```python
from build123d import *

# Parameters (mm, degrees)
CYLINDER_R        = 8
CYLINDER_DEPTH    = 5
CYLINDER001_R     = 2.5
CYLINDER001_DEPTH = 10
CHAMFER_SIZE      = 0.2
SKETCH_R          = 7.171484
SKETCH_R_2        = 3.208205
POCKET_DEPTH      = 0.3
SKETCH001_R       = 7.114293
SKETCH001_R_2     = 3.634589
POCKET001_DEPTH   = 0.3
CHAMFER001_SIZE   = 0.1


with BuildPart() as part:
    # Cylinder → Cylinder (join)
    with BuildSketch(Plane.XY):
        Circle(CYLINDER_R)
    extrude(amount=CYLINDER_DEPTH)

    # Cylinder001 → Cylinder001 (cut)
    with BuildSketch(Plane.XY):
        Circle(CYLINDER001_R)
    extrude(amount=CYLINDER001_DEPTH, mode=Mode.SUBTRACT)

    # Chamfer
    chamfer_edges = [part.edges().sort_by_distance(p)[0] for p in [
        (-8, 0, 5),
        (-8, 0, 0),
        (-2.5, 0, 5),
        (-2.5, 0, 0),
    ]]
    chamfer(chamfer_edges, length=CHAMFER_SIZE)

    # Sketch (on Face5 of Chamfer) → Pocket (cut)
    with BuildSketch(Plane.XY.offset(5)):
        Circle(SKETCH_R)
        Circle(SKETCH_R_2, mode=Mode.SUBTRACT)
    extrude(amount=-POCKET_DEPTH, mode=Mode.SUBTRACT)

    # Sketch001 (on Face4 of Pocket) → Pocket001 (cut)
    with BuildSketch(Plane(origin=(0, 0, 0), x_dir=(1, 0, 0), z_dir=(0, 0, -1))):
        Circle(SKETCH001_R)
        Circle(SKETCH001_R_2, mode=Mode.SUBTRACT)
    extrude(amount=-POCKET001_DEPTH, mode=Mode.SUBTRACT)

    # Chamfer001
    chamfer001_edges = [part.edges().sort_by_distance(p)[0] for p in [
        (-7.171484, 0, 5),
        (-7.114293, 0, 0),
    ]]
    chamfer(chamfer001_edges, length=CHAMFER001_SIZE)


solid = part.part
```
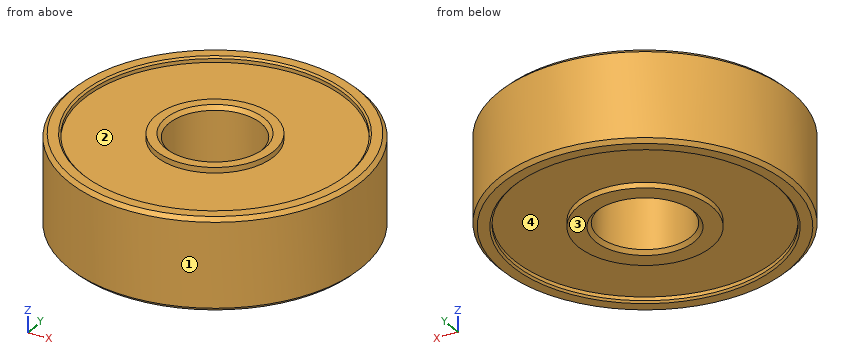
Check sheet for the modelled part. Datum: model origin and axes. Units: mm. Face numbers are marked on the shaded views. Round coordinates to 2 decimals unless told otherwise and drop trailing zeros. Order: outer loops, then holes, each group sorted by start corner. A loop starts at its lowest first (then second) coordinate and runs counter-clockwise, first axis right, second up. Notation, with made-up numbers: (58, 28) - (112, 28) arc R29 ccw to (112, 63) - close; hole circle Ø1 at (35, 32). An arc over 180 degrees is marked (long way). Answer as CSV lines item,"result". Start each with the question number.
1) Depth check by flat-ended pin: pin 1 (3 mm diameter, centred on x = 2.5, z = 2.5, fed in from -Y); pin 2 (3 mm diameter, centred on x = 0, y = 0, fed in from +Z); pin 3 (3 mm diameter, centred on x = -3, y = 4.5, fed in from +Z); pin 4 (1.5 mm diameter, centred on x = -2.5, z = 4.5, fed in from -Y). Enter the tip coordinate at first touch or a pass-through.
2) Scan lines: probe 1 along Y at (x, z) = (0, 3.85); probe 2 along Y at (x, z) = (0, 4.85); probe 3 along Z at (x, y) = (6.5, -2.5). Record each from-to range of solid material in increasing order.
3) Draft check along Y on the marked faces 1, 2, 3 and 4. Enter one of: +Y half, -Y half, draft (parallel to the pull), parting line (faces both ways), or undercut.
4) Section check A-A (z = 3.9). Record the cut outline in (x, y).
Determined:
1,pin 1,"y = -7.94"
1,pin 2,"through"
1,pin 3,"z = 4.7"
1,pin 4,"y = -7.81"
2,probe 1,"-8 to -2.5, 2.5 to 8"
2,probe 2,"-7.95 to -7.17, -3.21 to -2.55, 2.55 to 3.21, 7.17 to 7.95"
2,probe 3,"0.3 to 4.7"
3,face 1,"parting line"
3,face 2,"undercut"
3,face 3,"draft"
3,face 4,"undercut"
4,outline,"circle Ø16 at (0, 0); hole circle Ø5 at (0, 0)"
